from build123d import *

# Parameters (mm, degrees)
BOSS_EXTRUDE1_DEPTH      = 13
BOSS_EXTRUDE1_DEPTH_BACK = 3
SKETCH1_W                = 22.242116592
SKETCH1_H                = 30
SKETCH4_W                = 20.242116592
SKETCH4_H                = 12
CUT_EXTRUDE1_DEPTH       = 33
SKETCH3_W                = 1
SKETCH3_H                = 1
CUT_EXTRUDE2_DEPTH       = 2.1
SKETCH6_R                = 1.27
CUT_EXTRUDE3_DEPTH       = 3.1
BOSS_EXTRUDE3_DEPTH      = 29.459732878
SKETCH8_R                = 1
CUT_EXTRUDE4_DEPTH       = 39.644200609
LPATTERN1_COUNT          = 7
LPATTERN1_PITCH          = 3.71
FILLET2_R                = 1
OPTIONALCUT_DEPTH        = 39.644200609
OPTIONALCUT_DEPTH_BACK   = 39.644200609
SKETCH9_W                = 34.001532977
SKETCH9_H                = 12.141543576


with BuildPart() as part:
    # Sketch1 → Boss-Extrude1 (new, two sides: drawn at the far end of the back side and taken through both)
    with BuildSketch(Plane.XY.offset(-BOSS_EXTRUDE1_DEPTH_BACK)):
        with Locations((10.030822696, 14.459732878)):
            Rectangle(SKETCH1_W, SKETCH1_H)
    extrude(amount=BOSS_EXTRUDE1_DEPTH + BOSS_EXTRUDE1_DEPTH_BACK)

    # Sketch4 → Cut-Extrude1 (cut)
    with BuildSketch(Plane(origin=(0, 0, 0), x_dir=(1, 0, 0), z_dir=(0, 1, 0))):
        with Locations((10.030822696, -6)):
            Rectangle(SKETCH4_W, SKETCH4_H)
    extrude(amount=CUT_EXTRUDE1_DEPTH, mode=Mode.SUBTRACT)

    # Sketch3 → Cut-Extrude2 (cut)
    with BuildSketch(Plane.XY):
        with Locations((11.976170858, 3.750395558)):
            Rectangle(SKETCH3_W, SKETCH3_H)
        with Locations((8.476170858, 3.750395558)):
            Rectangle(SKETCH3_W, SKETCH3_H)
    extrude(amount=-CUT_EXTRUDE2_DEPTH, mode=Mode.SUBTRACT)

    # Sketch6 → Cut-Extrude3 (cut)
    with BuildSketch(Plane(origin=(0, 0, -3), x_dir=(-1, 0, 0), z_dir=(0, 0, -1))):
        with Locations((-17.651880992, 25.283129292)):
            Circle(SKETCH6_R)
        with Locations((-2.4097644, 25.283129292)):
            Circle(SKETCH6_R)
        with Locations((-17.751880992, 2.54676855)):
            Circle(SKETCH6_R)
        with Locations((-2.5097644, 2.54676855)):
            Circle(SKETCH6_R)
    extrude(amount=-CUT_EXTRUDE3_DEPTH, mode=Mode.SUBTRACT)

    # Sketch7 → Boss-Extrude3 (add)
    with BuildSketch(Plane(origin=(0, 0, 0), x_dir=(1, 0, 0), z_dir=(0, 1, 0))):
        Polygon((1.030822696, 3), (19.030822696, 3), (21.365822696, 7.044338636), (19.030822696, 11.088677271), (1.030822696, 11.088677271), (-1.304177304, 7.044338636), align=None)
    extrude(amount=BOSS_EXTRUDE3_DEPTH)

    # Sketch8 → Cut-Extrude4 (cut, symmetric)
    with BuildSketch(Plane(origin=(0, 0, 0), x_dir=(0, 0, -1), z_dir=(1, 0, 0))):
        with Locations(Location((5.1, 25.749732878, 0), (0, 0, 180))):
            Circle(SKETCH8_R)
    cut_extrude4 = extrude(amount=CUT_EXTRUDE4_DEPTH, both=True, mode=Mode.SUBTRACT)

    # LPattern1: Cut-Extrude4 ×7
    with Locations(*[(0, -i * LPATTERN1_PITCH, 0) for i in range(1, LPATTERN1_COUNT)]):
        add(cut_extrude4, mode=Mode.SUBTRACT)

    # Fillet2
    # the kernel refuses this fillet: 1 mm, written as the material it takes off along each edge
    with BuildSketch(Plane(origin=(20.151880992, 0.459732878, -2), x_dir=(0, 0, -1), z_dir=(1, 0, 0))) as fillet2_piece_1_section:
        Polygon((0, 0), (FILLET2_R * 1.02, 0), (FILLET2_R * 1.02, -FILLET2_R * 1.02), (0, -FILLET2_R * 1.02), align=None)
    fillet2_piece_1 = extrude(amount=FILLET2_R * 1.02, mode=Mode.PRIVATE)
    fillet2_piece_1 = fillet2_piece_1 - Plane(origin=(20.151880992, 0.459732878, -2), x_dir=(0, 0.7071067811865475, 0.7071067811865475), z_dir=(1, 0, 0)) * Sphere(FILLET2_R, mode=Mode.PRIVATE)
    add(fillet2_piece_1, mode=Mode.SUBTRACT)
    with BuildSketch(Plane(origin=(-0.0902356, 0.459732878, -2), x_dir=(0, 0, -1), z_dir=(-1, 0, 0))) as fillet2_piece_2_section:
        Polygon((0, 0), (FILLET2_R * 1.02, 0), (FILLET2_R * 1.02, FILLET2_R * 1.02), (0, FILLET2_R * 1.02), align=None)
    fillet2_piece_2 = extrude(amount=FILLET2_R * 1.02, mode=Mode.PRIVATE)
    fillet2_piece_2 = fillet2_piece_2 - Plane(origin=(-0.0902356, 0.459732878, -2), x_dir=(0, 0.7071067811865475, 0.7071067811865475), z_dir=(-1, 0, 0)) * Sphere(FILLET2_R, mode=Mode.PRIVATE)
    add(fillet2_piece_2, mode=Mode.SUBTRACT)
    with BuildSketch(Plane(origin=(20.151880992, 0.459732878, 12), x_dir=(1, 0, 0), z_dir=(0, 0, 1))) as fillet2_piece_3_section:
        Polygon((0, 0), (FILLET2_R * 1.02, 0), (FILLET2_R * 1.02, -FILLET2_R * 1.02), (0, -FILLET2_R * 1.02), align=None)
    fillet2_piece_3 = extrude(amount=FILLET2_R * 1.02, mode=Mode.PRIVATE)
    fillet2_piece_3 = fillet2_piece_3 - Plane(origin=(20.151880992, 0.459732878, 12), x_dir=(-0.7071067811865476, 0.7071067811865475, 0), z_dir=(0, 0, 1)) * Sphere(FILLET2_R, mode=Mode.PRIVATE)
    add(fillet2_piece_3, mode=Mode.SUBTRACT)
    with BuildSketch(Plane(origin=(-0.0902356, 0.459732878, 12), x_dir=(0, -1, 0), z_dir=(0, 0, 1))) as fillet2_piece_4_section:
        Polygon((0, 0), (FILLET2_R * 1.02, 0), (FILLET2_R * 1.02, -FILLET2_R * 1.02), (0, -FILLET2_R * 1.02), align=None)
    fillet2_piece_4 = extrude(amount=FILLET2_R * 1.02, mode=Mode.PRIVATE)
    fillet2_piece_4 = fillet2_piece_4 - Plane(origin=(-0.0902356, 0.459732878, 12), x_dir=(0.7071067811865475, 0.7071067811865477, 0), z_dir=(0, 0, 1)) * Sphere(FILLET2_R, mode=Mode.PRIVATE)
    add(fillet2_piece_4, mode=Mode.SUBTRACT)
    with BuildSketch(Plane(origin=(-0.0902356, 28.459732878, 12), x_dir=(-1, 0, 0), z_dir=(0, 1, 0))) as fillet2_piece_5_section:
        Polygon((0, 0), (FILLET2_R * 1.02, 0), (FILLET2_R * 1.02, FILLET2_R * 1.02), (0, FILLET2_R * 1.02), align=None)
    fillet2_piece_5 = extrude(amount=FILLET2_R * 1.02, mode=Mode.PRIVATE)
    fillet2_piece_5 = fillet2_piece_5 - Plane(origin=(-0.0902356, 28.459732878, 12), x_dir=(0.7071067811865475, 0, -0.7071067811865475), z_dir=(0, 1, 0)) * Sphere(FILLET2_R, mode=Mode.PRIVATE)
    add(fillet2_piece_5, mode=Mode.SUBTRACT)
    with BuildSketch(Plane(origin=(20.151880992, 28.459732878, 12), x_dir=(0, 0, 1), z_dir=(0, 1, 0))) as fillet2_piece_6_section:
        Polygon((0, 0), (FILLET2_R * 1.02, 0), (FILLET2_R * 1.02, FILLET2_R * 1.02), (0, FILLET2_R * 1.02), align=None)
    fillet2_piece_6 = extrude(amount=FILLET2_R * 1.02, mode=Mode.PRIVATE)
    fillet2_piece_6 = fillet2_piece_6 - Plane(origin=(20.151880992, 28.459732878, 12), x_dir=(-0.7071067811865475, 0, -0.7071067811865475), z_dir=(0, 1, 0)) * Sphere(FILLET2_R, mode=Mode.PRIVATE)
    add(fillet2_piece_6, mode=Mode.SUBTRACT)
    with BuildSketch(Plane(origin=(20.151880992, -0.540267122, -3), x_dir=(0, 1, 0), z_dir=(-1, 0, 0))) as fillet2_piece_7_section:
        with BuildLine():
            CenterArc((FILLET2_R, -FILLET2_R), FILLET2_R, 90, 90)
            Line((0, -FILLET2_R), (0, 0))
            Line((0, 0), (FILLET2_R, 0))
        make_face()
    fillet2_piece_7 = extrude(amount=20.242116592, mode=Mode.PRIVATE)
    fillet2_piece_7 = split(fillet2_piece_7, bisect_by=Plane(origin=(19.153997777, 0.112957923, -3.213345499), z_dir=(0.8660254037844363, 0, 0.5000000000000041)), keep=Keep.TOP, mode=Mode.PRIVATE)
    add(fillet2_piece_7, mode=Mode.SUBTRACT)
    with BuildSketch(Plane(origin=(20.151880992, -0.540267122, -3), x_dir=(0, 1, 0), z_dir=(-1, 0, 0))) as fillet2_piece_8_section:
        with BuildLine():
            CenterArc((FILLET2_R, -FILLET2_R), FILLET2_R, 90, 90)
            Line((0, -FILLET2_R), (0, 0))
            Line((0, 0), (FILLET2_R, 0))
        make_face()
    fillet2_piece_8 = extrude(amount=20.242116592, mode=Mode.PRIVATE)
    fillet2_piece_8 = split(fillet2_piece_8, bisect_by=Plane(origin=(10.030822696, 0, -2.762798919), z_dir=(0, -1, 0)), keep=Keep.TOP, mode=Mode.PRIVATE)
    add(fillet2_piece_8, mode=Mode.SUBTRACT)
    with BuildSketch(Plane(origin=(20.151880992, -0.540267122, -3), x_dir=(0, 1, 0), z_dir=(-1, 0, 0))) as fillet2_piece_9_section:
        with BuildLine():
            CenterArc((FILLET2_R, -FILLET2_R), FILLET2_R, 90, 90)
            Line((0, -FILLET2_R), (0, 0))
            Line((0, 0), (FILLET2_R, 0))
        make_face()
    fillet2_piece_9 = extrude(amount=20.242116592, mode=Mode.PRIVATE)
    fillet2_piece_9 = split(fillet2_piece_9, bisect_by=Plane(origin=(0.907647615, 0.112957923, -3.213345499), z_dir=(-0.8660254037844362, 0, 0.5000000000000044)), keep=Keep.TOP, mode=Mode.PRIVATE)
    add(fillet2_piece_9, mode=Mode.SUBTRACT)
    with BuildSketch(Plane(origin=(20.151880992, -0.540267122, 13), x_dir=(0, 1, 0), z_dir=(-1, 0, 0))) as fillet2_piece_10:
        with BuildLine():
            CenterArc((FILLET2_R, FILLET2_R), FILLET2_R, 180, 90)
            Line((0, FILLET2_R), (0, 0))
            Line((0, 0), (FILLET2_R, 0))
        make_face()
    extrude(amount=20.242116592, mode=Mode.SUBTRACT)
    with BuildSketch(Plane(origin=(-1.0902356, 0.459732878, -3), x_dir=(1, 0, 0), z_dir=(0, 1, 0))) as fillet2_piece_11:
        with BuildLine():
            CenterArc((FILLET2_R, -FILLET2_R), FILLET2_R, 90, 90)
            Line((0, -FILLET2_R), (0, 0))
            Line((0, 0), (FILLET2_R, 0))
        make_face()
    extrude(amount=31.5, mode=Mode.SUBTRACT)
    with BuildSketch(Plane(origin=(-1.0902356, 29.459732878, -5.5), x_dir=(1, 0, 0), z_dir=(0, 0, 1))) as fillet2_piece_12_section:
        with BuildLine():
            CenterArc((FILLET2_R, -FILLET2_R), FILLET2_R, 90, 90)
            Line((0, -FILLET2_R), (0, 0))
            Line((0, 0), (FILLET2_R, 0))
        make_face()
    fillet2_piece_12 = extrude(amount=17.5, mode=Mode.PRIVATE)
    fillet2_piece_12 = split(fillet2_piece_12, bisect_by=Plane(origin=(1.20591916, 29.236364939, -2.696724029), z_dir=(-0.8660254037844362, 0, 0.5000000000000044)), keep=Keep.TOP, mode=Mode.PRIVATE)
    add(fillet2_piece_12, mode=Mode.SUBTRACT)
    with BuildSketch(Plane(origin=(-1.0902356, 0.459732878, 13), x_dir=(1, 0, 0), z_dir=(0, 1, 0)), Plane(origin=(21.151880992, 28.459732878, 13), x_dir=(-1, 0, 0), z_dir=(0, -1, 0))) as fillet2_piece_13:
        with BuildLine():
            CenterArc((FILLET2_R, FILLET2_R), FILLET2_R, 180, 90)
            Line((0, FILLET2_R), (0, 0))
            Line((0, 0), (FILLET2_R, 0))
        make_face()
    extrude(amount=28, mode=Mode.SUBTRACT)
    with BuildSketch(Plane(origin=(-1.0902356, -0.540267122, -2), x_dir=(0, 1, 0), z_dir=(0, 0, 1)), Plane(origin=(21.151880992, -0.540267122, 12), x_dir=(0, 1, 0), z_dir=(0, 0, -1))) as fillet2_piece_14:
        with BuildLine():
            CenterArc((FILLET2_R, -FILLET2_R), FILLET2_R, 90, 90)
            Line((0, -FILLET2_R), (0, 0))
            Line((0, 0), (FILLET2_R, 0))
        make_face()
    extrude(amount=14, mode=Mode.SUBTRACT)
    with BuildSketch(Plane(origin=(21.151880992, 31.959732878, -3), x_dir=(0, 0, 1), z_dir=(0, -1, 0))) as fillet2_piece_15:
        with BuildLine():
            CenterArc((FILLET2_R, FILLET2_R), FILLET2_R, 180, 90)
            Line((0, FILLET2_R), (0, 0))
            Line((0, 0), (FILLET2_R, 0))
        make_face()
    extrude(amount=31.5, mode=Mode.SUBTRACT)
    with BuildSketch(Plane(origin=(21.151880992, 29.459732878, 12), x_dir=(-1, 0, 0), z_dir=(0, 0, -1))) as fillet2_piece_16_section:
        with BuildLine():
            CenterArc((FILLET2_R, -FILLET2_R), FILLET2_R, 90, 90)
            Line((0, -FILLET2_R), (0, 0))
            Line((0, 0), (FILLET2_R, 0))
        make_face()
    fillet2_piece_16 = extrude(amount=17.5, mode=Mode.PRIVATE)
    fillet2_piece_16 = split(fillet2_piece_16, bisect_by=Plane(origin=(15.608130968, 29.236364939, 2.928275971), z_dir=(0.8660254037844363, 0, 0.5000000000000041)), keep=Keep.TOP, mode=Mode.PRIVATE)
    add(fillet2_piece_16, mode=Mode.SUBTRACT)
    with BuildSketch(Plane(origin=(-0.0902356, 29.459732878, 13), x_dir=(0, 0, -1), z_dir=(1, 0, 0))) as fillet2_piece_17:
        with BuildLine():
            CenterArc((FILLET2_R, -FILLET2_R), FILLET2_R, 90, 90)
            Line((0, -FILLET2_R), (0, 0))
            Line((0, 0), (FILLET2_R, 0))
        make_face()
    extrude(amount=20.242116592, mode=Mode.SUBTRACT)

    # Sketch9 → OptionalCut (cut, two sides: drawn at the far end of the back side and taken through both)
    with BuildSketch(Plane(origin=(0, 0, 0), x_dir=(1, 0, 0), z_dir=(0, 1, 0)).offset(-OPTIONALCUT_DEPTH_BACK)):
        with Locations((10.877994957, -10.695825978)):
            Rectangle(SKETCH9_W, SKETCH9_H)
    extrude(amount=OPTIONALCUT_DEPTH + OPTIONALCUT_DEPTH_BACK, mode=Mode.SUBTRACT)


solid = part.part
Build history of the part. All positions in model axes, mm. A direction names the side the tool comes from. Give positions to 0.01 mm unless a question says otherwise; leave off trailing zeros. Write each loop counter-clockwise with the first axis right and the second up, starting at its lowest first coordinate (ties: lowest second). Pieces come first, ordered by that corner, then holes. Notation, with made-up numbers: (32.25, -25.75) - (63.25, -25.75) arc R17 cw to (63.25, 0.25) - close; hole circle Ø3 at (-22.75, -20.5). An arc over 180 degrees is marked (long way). Use one line per item in the form item = value. Start each with the question number.
1. Band-saw the part on B-B on y = 5. Write the cut outline in (x, z).
2. Band-saw the part on C-C on x = 7.25. Write the cut outline in (y, z), plus the area to 3 significant figures.
3. Drop flat-ended pins along their axis: pin 1 Ø1.1 at (x, y) = (12, 3.5) entering from +Z; pin 2 Ø3.5 at (y, z) = (12.5, 1) entering from -X; pin 3 Ø3 at (y, z) = (7.2, -5.1) entering from +X. Give the stop position or say it passes through.
4. 3-axis set-ups, long thin cutter, end or side, ignore diameter. For faces 1 (the face through (-0.09, 15, 2)), 2 (the face through (2, 25, -3)), 3 (the face through (20.851, 15.163, -2.715)), 4 (the face through (10, -0.54, 1)): which of +Z, -Z, +X, -X, +Y, -Y reach the whole face in a straight line?
5. Two-plate mould, pull along X, no slides. Class faces 5 (the face through (8.5, 3.8, -2.1)), 6 (the face through (-1.09, 14, 1)), 7 (the face through (8.5, 4.25, -1)), 8 (the face through (10.2, 18.3, -6.1)): released by +X, released by -X, zero draft, split by the parting line, or undercut.
6. Band-saw the part on D-D on z = -7.75. Write the cut outline in (x, y), plus the area to 3 significant figures.
7. Band-saw the part on A-A on z = 1.5. Write the cut outline in (x, y).
8. Probe line 1 (X direction, y = 20.75, z = 0.25); line 2 (Z direction, x = 7.25, y = 25.75); line 3 (Y direction, x = 3.25, z = -7.75). List the from-to ranges inside material, lowest first. Write a range as [from, to].
Conclusion:
q1.outline = (-1.3, -7.04) - (1.03, -11.09) - (19.03, -11.09) - (21.37, -7.04) - (19.03, -3) - (20.15, -3) arc R1 ccw to (21.15, -2) - (21.15, 4.63) - (20.15, 4.63) - (20.15, 0) - (-0.09, 0) - (-0.09, 4.63) - (-1.09, 4.63) - (-1.09, -2) arc R1 ccw to (-0.09, -3) - (1.03, -3) - close
q2.outline = (-0.54, -2) arc R1 ccw to (0, -2.89) - (0, -11.09) - (29.46, -11.09) - (29.46, 0) - (0, 0) - (0, 4.63) - (-0.54, 4.63) - close; hole circle Ø2 at (3.49, -5.1); hole circle Ø2 at (7.2, -5.1); hole circle Ø2 at (10.91, -5.1); hole circle Ø2 at (14.62, -5.1); hole circle Ø2 at (18.33, -5.1); hole circle Ø2 at (22.04, -5.1); hole circle Ø2 at (25.75, -5.1)
q2.area = 309 mm²
q3.pin_1 = 0
q3.pin_2 = -1.09
q3.pin_3 = 21.11
q4.face_1 = +Z, +Y
q4.face_2 = +Z
q4.face_3 = +X, +Y, -Y
q4.face_4 = +Z, -Z, +X, -X, -Y
q5.face_5 = undercut
q5.face_6 = released by -X
q5.face_7 = undercut
q5.face_8 = zero draft
q6.outline = (-0.9, 0) - (20.96, 0) - (20.96, 29.46) - (-0.9, 29.46) - close
q6.area = 644 mm²
q7.outline = (-1.09, 0.46) arc R1 ccw to (-0.09, -0.54) - (20.15, -0.54) arc R1 ccw to (21.15, 0.46) - (21.15, 28.46) arc R1 ccw to (20.15, 29.46) - (20.15, 0) - (-0.09, 0) - (-0.09, 29.46) arc R1 ccw to (-1.09, 28.46) - close
q8.line_1 = [-1.09, -0.09], [20.15, 21.15]
q8.line_2 = [-11.09, -6.1], [-4.1, 0]
q8.line_3 = [0, 29.46]
